Geometry check sheet. Reference: the model listing, model coordinates, mm. A direction names the side the tool comes from. Coordinates: 2 decimals unless noted, no trailing zeros. Write each loop counter-clockwise with the first axis right and the second up, starting at its lowest first coordinate (ties: lowest second). Pieces come first, ordered by that corner, then holes. Notation, with made-up numbers: (3.5, -1) -> (18.5, -1) arc R33 cw to (18.5, 27) -> close; hole circle Ø8 at (54, 14). An arc over 180 degrees is marked (long way). Use a Markdown table: item, result.
```python
from build123d import *

# Parameters (mm, degrees)
F0_W     = 37.75
F0_H     = 24.5
F1_DEPTH = 0.7
F2_W     = 6
F2_H     = 6
F3_DEPTH = 1
F4_W     = 3
F4_H     = 3
F5_DEPTH = 1
F6_R     = 1
F7_DEPTH = 1
F8_W     = 7.5
F8_H     = 6
F9_DEPTH = 2


with BuildPart() as f1:
    # F0 (on Top) → F1 (new body)
    with BuildSketch(Plane.XY):
        with Locations((18.875, 12.25)):
            Rectangle(F0_W, F0_H)
    extrude(amount=F1_DEPTH)

    # F2 (on face) → F3 (join)
    with BuildSketch(Plane.XY.offset(0.7)):
        with Locations((9.25, 3.25)):
            Rectangle(F2_W, F2_H)
        with Locations((18.75, 3.25)):
            Rectangle(F2_W, F2_H)
        with Locations((28.25, 3.25)):
            Rectangle(F2_W, F2_H)
    extrude(amount=F3_DEPTH)

    # F4 (on face) → F5 (join)
    with BuildSketch(Plane.XY.offset(0.7)):
        with Locations((9.25, 13.142036)):
            Rectangle(F4_W, F4_H)
        with Locations((18.75, 13.142036)):
            Rectangle(F4_W, F4_H)
        with Locations((28.25, 13.142036)):
            Rectangle(F4_W, F4_H)
    extrude(amount=F5_DEPTH)

    # F6 (on face) → F7 (join)
    with BuildSketch(Plane.XY.offset(1.7)):
        with Locations((9.25, 13.142036)):
            Circle(F6_R)
        with Locations((18.75, 13.046024)):
            Circle(F6_R)
        with Locations((28.25, 13.203288)):
            Circle(F6_R)
    extrude(amount=F7_DEPTH)

    # F8 (on face) → F9 (join)
    with BuildSketch(Plane.XY.offset(0.7)):
        with Locations((18.75, 23)):
            Rectangle(F8_W, F8_H)
    extrude(amount=F9_DEPTH)


solid = f1.part
```
Item 1: Mould release check, pull along Y, two halves, no side actions. Record for faces 4 (the flat face through (9, 6.25, 1)), 5 (the flat face through (7.75, 13, 1)), 6 (the flat face through (9, 14.642, 1)): +Y half, -Y half, draft (parallel to the pull), parting line (faces both ways), or undercut.
Answer block:
| item | result |
|---|---|
| face 4 | undercut |
| face 5 | draft |
| face 6 | +Y half |
Item 2: Section check B-B on y = 5.5. Record the boundary of the cut face in (x, z).
Answer block:
| item | result |
|---|---|
| outline | (0, 0) -> (37.75, 0) -> (37.75, 0.7) -> (31.25, 0.7) -> (31.25, 1.7) -> (25.25, 1.7) -> (25.25, 0.7) -> (21.75, 0.7) -> (21.75, 1.7) -> (15.75, 1.7) -> (15.75, 0.7) -> (12.25, 0.7) -> (12.25, 1.7) -> (6.25, 1.7) -> (6.25, 0.7) -> (0, 0.7) -> close |
Item 3: Section check C-C on x = 9.25. Record the boundary of the cut face in (y, z), then the cut area to 4 significant figures.
Answer block:
| item | result |
|---|---|
| outline | (0, 0) -> (24.5, 0) -> (24.5, 0.7) -> (14.64, 0.7) -> (14.64, 1.7) -> (14.14, 1.7) -> (14.14, 2.7) -> (12.14, 2.7) -> (12.14, 1.7) -> (11.64, 1.7) -> (11.64, 0.7) -> (6.25, 0.7) -> (6.25, 1.7) -> (0.25, 1.7) -> (0.25, 0.7) -> (0, 0.7) -> close |
| area | 28.15 mm^2 |
Item 4: Tool access check on faces 1 (the flat face through (10.75, 13, 1)), 2 (the flat face through (19, 11.642, 1)), 3 (the flat face through (20.25, 13, 1)). Record the directions out of +Z, -Z, +X, -X, +Y, -Y that give a thin tool (end or side, any length) a straight path to the whole face; none if there is none.
Answer block:
| item | result |
|---|---|
| face 1 | +Z, +Y |
| face 2 | +Z, +X, -X |
| face 3 | +Z |
Item 5: Thickness scan on L1, parallel to X at y = 24.5, z = 1.7; L2, parallel to Z at x = 19.5, y = 8.75; L3, parallel to X at y = 12.75, z = 1.8. Record the ranges inside material, lowest first. Write a range as [from, to].
Answer block:
| item | result |
|---|---|
| L1 | x = [15, 22.5] |
| L2 | z = [0, 0.7] |
| L3 | x = [8.33, 10.17], [17.79, 19.71], [27.36, 29.14] |
Item 6: Depth check by flat-ended pin: P1, Ø0.5, axis at y = 14, z = 1.5, coming from the -X side; P2, Ø5, axis at x = 17.5, y = 2.5, coming from the +Z side; P3, Ø0.5, axis at y = 13, z = 1, coming from the +X side. Enter the tip coordinate at first touch or a pass-through.
Answer block:
| item | result |
|---|---|
| P1 | stops at x = 7.75 |
| P2 | stops at z = 1.7 |
| P3 | stops at x = 29.75 |
Item 7: Section check A-A on x = 18.75. Record the boundary of the cut face in (y, z), then the cut area to 4 significant figures.
Answer block:
| item | result |
|---|---|
| outline | (0, 0) -> (24.5, 0) -> (24.5, 0.7) -> (26, 0.7) -> (26, 2.7) -> (20, 2.7) -> (20, 0.7) -> (14.64, 0.7) -> (14.64, 1.7) -> (14.05, 1.7) -> (14.05, 2.7) -> (12.05, 2.7) -> (12.05, 1.7) -> (11.64, 1.7) -> (11.64, 0.7) -> (6.25, 0.7) -> (6.25, 1.7) -> (0.25, 1.7) -> (0.25, 0.7) -> (0, 0.7) -> close |
| area | 40.15 mm^2 |
